Input: part model. Units: mm. Frame: model coordinates. A direction names the side the tool comes from. Round coordinates to 2 decimals unless told otherwise and drop trailing zeros. Loops run counter-clockwise (first coordinate to the right, second up) from the corner with the lowest first, then second, coordinate; pieces in that order, holes last. Notation, with made-up numbers: M 44.25,-24.5 L 57.25,-24.5 A8 ccw 57.25,-18.5 Z; hole C -33,69 d6. An arc over 180 degrees is marked long. Put each result on its own line as item: value. Start each with the question number.
1) Section D-D on y = 56.5. Output: boundary loops of the cut face in (x, z), plus the area to 3 significant figures.
2) Pin query (flat end, axial travel): pin 1 (18.5 mm diameter, centred on x = 80.5, y = 24, fed in from -Z); pin 2 (2.5 mm diameter, centred on y = 47, z = -8.5, fed in from -X); pin 3 (3 mm diameter, centred on x = 68.5, y = 5.5, fed in from +Z); pin 4 (7 mm diameter, centred on x = 58.5, z = -7.5, fed in from +Y). Return the tip coordinate at first contact, or that it passes through.
3) Section B-B on x = 68.5. Output: boundary loops of the cut face in (y, z).
4) Section C-C on y = 21. Output: boundary loops of the cut face in (x, z), plus the area to 4 significant figures.
5) Reachability of faces 1 (the face through (69.33, 38.22, -11)), 2 (the face through (70.65, 33.127, -6.944)), 3 (the face through (105, 31, -6)), 4 (the face through (57, 5, -8)), 5 (the face through (47, 52, -8)) from +Z, -Z, +X, -X, +Y, -Y: full face, straight path, thin tool, end or side. Return the list, or none.
6) Section A-A on z = -4.5. State how many separate pieces and enclosed holes the cut face has, plus the area to 3 significant figures.
7) Draft query along Y for faces 6 (the face through (66.1, 3.7, -3.9)), 7 (the face through (84, 50, -8)), 8 (the face through (44, 42, -8)). Return one class per face: +Y half, -Y half, draft (parallel to the pull), parting line (faces both ways), or undercut.
8) Line query: probe 1 along Y at (x, z) = (94, -7.5); probe 2 along Y at (x, z) = (8, -5); probe 3 along X at (y, z) = (40, -11.5). Output: solid intervals per line, ascending.
from build123d import *

# Parameters (mm, degrees)
SKETCH_R        = 2.25
SKETCH_R_2      = 11.25
SKETCH_R_3      = 1.75
PAD_DEPTH       = 12
POCKET_DEPTH    = 9
SKETCH002_R     = 4
PAD001_DEPTH    = 8
SKETCH003_R     = 3
POCKET001_DEPTH = 8
SKETCH004_R     = 1.75
POCKET002_DEPTH = 5


with BuildPart() as pocket_belt_path:
    # Sketch → Pad (new body)
    with BuildSketch(Plane.XY):
        Polygon((0, 0), (105, 0), (105, 62), (20, 62), (20, 42), (0, 42), align=None)
        with Locations((38, 10)):
            Circle(SKETCH_R, mode=Mode.SUBTRACT)
        with Locations((33, 35)):
            Circle(SKETCH_R, mode=Mode.SUBTRACT)
        with Locations((84, 21)):
            Circle(SKETCH_R_2, mode=Mode.SUBTRACT)
        with Locations((68.5, 36.5)):
            Circle(SKETCH_R_3, mode=Mode.SUBTRACT)
        with Locations((99.5, 36.5)):
            Circle(SKETCH_R_3, mode=Mode.SUBTRACT)
        with Locations((68.5, 5.5)):
            Circle(SKETCH_R_3, mode=Mode.SUBTRACT)
        with Locations((99.5, 5.5)):
            Circle(SKETCH_R_3, mode=Mode.SUBTRACT)
        with Locations((10, 30)):
            Circle(SKETCH_R, mode=Mode.SUBTRACT)
        with Locations((10, 15)):
            Circle(SKETCH_R, mode=Mode.SUBTRACT)
        with Locations((42, 52)):
            Circle(SKETCH_R, mode=Mode.SUBTRACT)
        with Locations((94, 52)):
            Circle(SKETCH_R, mode=Mode.SUBTRACT)
        with Locations((55, 5)):
            Circle(SKETCH_R_3, mode=Mode.SUBTRACT)
        with BuildLine():
            Line((58.75, 25.000001), (58.75, 40))
            ThreePointArc((58.75, 40), (56.5, 42.25), (54.25, 39.999999))
            Line((54.25, 25), (54.25, 39.999999))
            ThreePointArc((54.25, 25), (56.5, 22.75), (58.75, 25.000001))
        make_face(mode=Mode.SUBTRACT)
    extrude(amount=PAD_DEPTH)

    # Sketch001 → Pocket (cut)
    with BuildSketch(Plane.XY.offset(12)):
        with BuildLine():
            ThreePointArc((41.485277, 42), (39.015593, 44.209375), (35.999996, 45.583005))
            Line((35.999996, 67), (35.999996, 45.583005))
            Line((20, 67), (35.999996, 67))
            Line((20, -1), (20, 67))
            Line((20, -1), (48.252269, -1))
            Line((48.252269, 11), (48.252269, -1))
            Line((48.252269, 11), (70.252269, 11))
            ThreePointArc((70.252269, 11), (71.759618, 9.202833), (73.499996, 7.630258))
            Line((73.499996, 7.630258), (73.499996, -1))
            Line((73.499996, -1), (93.499996, -1))
            Line((93.499996, -1), (93.499996, 6.902128))
            ThreePointArc((93.499996, 6.902128), (95.574295, 8.548671), (97.367695, 10.497399))
            Line((105.499996, 10.497399), (97.367695, 10.497399))
            Line((105.499996, 30.497399), (105.499996, 10.497399))
            Line((98.099621, 30.497399), (105.499996, 30.497399))
            ThreePointArc((98.099621, 30.497399), (91.98574, 36.007594), (83.999996, 38))
            Line((83.999996, 38), (83.999996, 67))
            Line((83.999996, 67), (46.999996, 67))
            Line((46.999996, 67), (46.999996, 42))
            Line((41.485277, 42), (46.999996, 42))
        make_face()
    extrude(amount=-POCKET_DEPTH, mode=Mode.SUBTRACT)


with BuildPart() as pocket002:
    # Part__Mirroring: instance of Pocket belt path
    add(pocket_belt_path.part.mirror(Plane(origin=(52.5, 31, 0), x_dir=(0, 1, 0), z_dir=(0, 0, 1))))

    # Sketch002 → Pad001 (new body)
    with BuildSketch(Plane(origin=(0, 0, -3), x_dir=(1, 0, 0), z_dir=(0, 0, -1))):
        with Locations((68.5, -36.5)):
            Circle(SKETCH002_R)
    extrude(amount=PAD001_DEPTH)

    # Sketch003 → Pocket001 (cut)
    with BuildSketch(Plane.XY):
        with Locations((55, 5)):
            Circle(SKETCH003_R)
        with Locations((68.5, 36.5)):
            Circle(SKETCH003_R)
        with Locations((68.5, 5.5)):
            Circle(SKETCH003_R)
        with Locations((99.5, 36.5)):
            Circle(SKETCH003_R)
        with Locations((99.5, 5.5)):
            Circle(SKETCH003_R)
    extrude(amount=-POCKET001_DEPTH, mode=Mode.SUBTRACT)

    # Sketch004 → Pocket002 (cut)
    with BuildSketch(Plane.XY.offset(-8)):
        with Locations((68.5, 36.5)):
            Circle(SKETCH004_R)
    extrude(amount=-POCKET002_DEPTH, mode=Mode.SUBTRACT)


solid = pocket002.part
Geometry results:
1. outline: M 20,-3 L 36,-3 L 36,-12 L 47,-12 L 47,-3 L 84,-3 L 84,-12 L 105,-12 L 105,0 L 20,0 Z
1. area: 543 mm²
2. pin 1: stops at z = -3
2. pin 2: stops at x = 36
2. pin 3: passes through
2. pin 4: stops at y = 11
3. outline: M 0,-12 L 3.75,-12 L 3.75,-8 L 2.5,-8 L 2.5,0 L 0,0 Z; M 7.25,-12 L 11,-12 L 11,-3 L 32.5,-3 L 32.5,-11 L 34.75,-11 L 34.75,-8 L 33.5,-8 L 33.5,0 L 8.5,0 L 8.5,-8 L 7.25,-8 Z; M 38.25,-11 L 40.5,-11 L 40.5,-3 L 62,-3 L 62,0 L 39.5,0 L 39.5,-8 L 38.25,-8 Z
4. outline: M 0,-12 L 20,-12 L 20,-3 L 72.75,-3 L 72.75,0 L 0,0 Z; M 95.25,-3 L 105,-3 L 105,0 L 95.25,0 Z
4. area: 427.5 mm²
5. face 1: -Z, +Y
5. face 2: -Z
5. face 3: +Z, -Z, +X, +Y, -Y
5. face 4: +Z
5. face 5: -Z, +Y, -Y
6. separate pieces: 6
6. enclosed holes: 9
6. area: 1,870 mm²
7. face 6: undercut
7. face 7: draft
7. face 8: -Y half
8. probe 1: y = 0 to 7.25, 34.75 to 49.75, 54.25 to 62
8. probe 2: y = 0 to 13.97, 16.03 to 28.97, 31.03 to 42
8. probe 3: x = 0 to 20, 84 to 105
